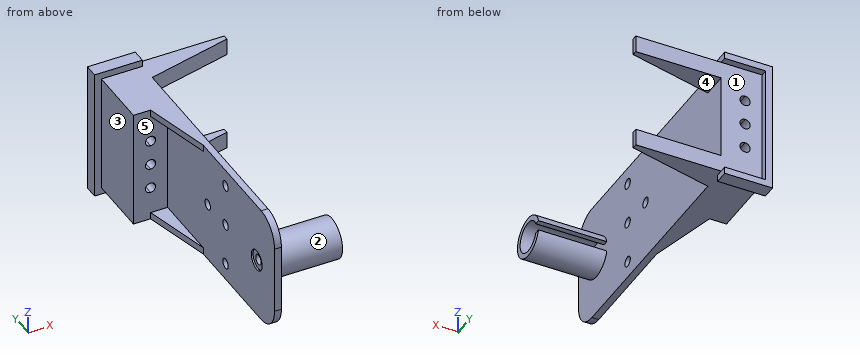
```python
from build123d import *

# Parameters (mm, degrees)
SALIENTE_EXTRUIR1_DEPTH      = 40
SALIENTE_EXTRUIR2_DEPTH      = 4
CROQUIS3_R                   = 3
CORTAR_EXTRUIR1_DEPTH        = 4
CROQUIS4_R                   = 6
CORTAR_EXTRUIR2_DEPTH        = 1
SALIENTE_EXTRUIR3_DEPTH      = 40
SALIENTE_EXTRUIR4_START      = 25
SALIENTE_EXTRUIR4_DEPTH      = 10
SALIENTE_EXTRUIR5_START      = -25
SALIENTE_EXTRUIR5_DEPTH      = 10
SALIENTE_EXTRUIR6_DEPTH      = 4
SALIENTE_EXTRUIR6_DEPTH_BACK = 4
SALIENTE_EXTRUIR6_START      = 140
SALIENTE_EXTRUIR7_START      = 31
SALIENTE_EXTRUIR7_DEPTH      = 4
SALIENTE_EXTRUIR8_START      = -31
SALIENTE_EXTRUIR8_DEPTH      = 4
CORTAR_EXTRUIR3_DEPTH        = 4
CORTAR_EXTRUIR4_DEPTH        = 4
CROQUIS22_R                  = 3
CORTAR_EXTRUIR5_DEPTH        = 4


with BuildPart() as part:
    # Croquis1 → Saliente-Extruir1 (new body)
    with BuildSketch(Plane(origin=(0, 0, 0), x_dir=(0, 0, -1), z_dir=(1, 0, 0))):
        with BuildLine():
            Line((3, 9), (3, 11.618950039))
            ThreePointArc((3, 11.618950039), (0, -12), (-3, 11.618950039))
            Line((-3, 11.618950039), (-3, 9))
            Line((-3, 9), (-3, 8.485281374))
            ThreePointArc((-3, 8.485281374), (0, -9), (3, 8.485281374))
            Line((3, 8.485281374), (3, 9))
        make_face()
    extrude(amount=SALIENTE_EXTRUIR1_DEPTH)

    # Croquis2 → Saliente-Extruir2 (add)
    with BuildSketch(Plane.ZY):
        Polygon((-35, 0), (-35, 140), (35, 140), (35, 0), (35, -20), (-35, -20), align=None)
    extrude(amount=SALIENTE_EXTRUIR2_DEPTH)

    # Croquis3 → Cortar-Extruir1 (cut)
    with BuildSketch(Plane(origin=(0, 0, 0), x_dir=(0, 0, -1), z_dir=(1, 0, 0))):
        Circle(CROQUIS3_R)
    extrude(amount=-CORTAR_EXTRUIR1_DEPTH, mode=Mode.SUBTRACT)

    # Croquis4 → Cortar-Extruir2 (cut)
    with BuildSketch(Plane.ZY.offset(4)):
        Circle(CROQUIS4_R)
    extrude(amount=-CORTAR_EXTRUIR2_DEPTH, mode=Mode.SUBTRACT)

    # Croquis6 → Saliente-Extruir3 (add)
    with BuildSketch(Plane(origin=(0, 140, 0), x_dir=(1, 0, 0), z_dir=(0, 1, 0))):
        with BuildLine():
            Line((-14, 30), (-14, 35))
            Line((-14, 35), (-24, 35))
            Line((-24, 35), (-24, -35))
            Line((-24, -35), (-14, -35))
            Line((-14, -35), (-14, -30))
            Line((-14, -30), (-14, -18))
            ThreePointArc((-14, -18), (-17, -15), (-14, -12))
            Line((-14, -12), (-14, -3))
            ThreePointArc((-14, -3), (-17, 0), (-14, 3))
            Line((-14, 3), (-14, 12))
            ThreePointArc((-14, 12), (-17, 15), (-14, 18))
            Line((-14, 18), (-14, 30))
        make_face()
        with BuildLine():
            Line((-4, 35), (-14, 35))
            Line((-14, 35), (-14, 30))
            Line((-14, 30), (-14, 18))
            ThreePointArc((-14, 18), (-11.878679656, 17.121320344), (-11, 15))
            ThreePointArc((-11, 15), (-11.878679656, 12.878679656), (-14, 12))
            Line((-14, 12), (-14, 3))
            ThreePointArc((-14, 3), (-11.878679656, 2.121320344), (-11, 0))
            ThreePointArc((-11, 0), (-11.878679656, -2.121320344), (-14, -3))
            Line((-14, -3), (-14, -12))
            ThreePointArc((-14, -12), (-11.878679656, -12.878679656), (-11, -15))
            ThreePointArc((-11, -15), (-11.878679656, -17.121320344), (-14, -18))
            Line((-14, -18), (-14, -30))
            Line((-14, -30), (-14, -35))
            Line((-14, -35), (-4, -35))
            Line((-4, -35), (-4, 35))
        make_face()
    extrude(amount=-SALIENTE_EXTRUIR3_DEPTH)

    # Croquis7 → Saliente-Extruir4 (add)
    with BuildSketch(Plane.XY.offset(SALIENTE_EXTRUIR4_START)):
        Polygon((0, 140), (50, 140), (50, 137), (0, 125), align=None)
    extrude(amount=SALIENTE_EXTRUIR4_DEPTH)

    # Croquis8 → Saliente-Extruir5 (add)
    with BuildSketch(Plane.XY.offset(SALIENTE_EXTRUIR5_START)):
        Polygon((0, 140), (50, 140), (50, 137), (0, 125), align=None)
    extrude(amount=-SALIENTE_EXTRUIR5_DEPTH)

    # Croquis9 → Saliente-Extruir6 (add, two sides: drawn at the far end of the back side and taken through both)
    with BuildSketch(Plane(origin=(0, 0, 0), x_dir=(1, 0, 0), z_dir=(0, 1, 0)).offset(SALIENTE_EXTRUIR6_START - SALIENTE_EXTRUIR6_DEPTH_BACK)):
        Polygon((0, 35), (0, 39), (-28, 39), (-28, -39), (-24, -39), (0, -39), (0, -35), (-24, -35), (-24, 35), align=None)
    extrude(amount=SALIENTE_EXTRUIR6_DEPTH + SALIENTE_EXTRUIR6_DEPTH_BACK)

    # Croquis16 → Saliente-Extruir7 (add)
    with BuildSketch(Plane.XY.offset(SALIENTE_EXTRUIR7_START)):
        Polygon((-14, 100), (-4, 60), (-4, 100), align=None)
    extrude(amount=SALIENTE_EXTRUIR7_DEPTH)

    # Croquis17 → Saliente-Extruir8 (add)
    with BuildSketch(Plane.XY.offset(SALIENTE_EXTRUIR8_START)):
        Polygon((-4, 100), (-14, 100), (-4, 60), align=None)
    extrude(amount=-SALIENTE_EXTRUIR8_DEPTH)

    # Croquis19 → Cortar-Extruir3 (cut)
    with BuildSketch(Plane.ZY.offset(4)):
        with BuildLine():
            Line((-35, -20), (-20, -20))
            ThreePointArc((-20, -20), (-30.606601718, -15.606601718), (-35, -5))
            Line((-35, -5), (-35, -20))
        make_face()
        with BuildLine():
            Line((35, -20), (20, -20))
            ThreePointArc((20, -20), (30.606601718, -15.606601718), (35, -5))
            Line((35, -5), (35, -20))
        make_face()
    extrude(amount=-CORTAR_EXTRUIR3_DEPTH, mode=Mode.SUBTRACT)

    # Croquis20 → Cortar-Extruir4 (cut)
    with BuildSketch(Plane.ZY.offset(4)):
        with BuildLine():
            ThreePointArc((-22, 35), (-25, 38), (-28, 35))
            Line((-28, 35), (-22, 35))
        make_face()
        with BuildLine():
            Line((-22, 35), (-28, 35))
            ThreePointArc((-28, 35), (-25, 32), (-22, 35))
        make_face()
        with BuildLine():
            ThreePointArc((3, 35), (0, 38), (-3, 35))
            Line((-3, 35), (3, 35))
        make_face()
        with BuildLine():
            Line((3, 35), (-3, 35))
            ThreePointArc((-3, 35), (0, 32), (3, 35))
        make_face()
        with BuildLine():
            ThreePointArc((22, 35), (25, 32), (28, 35))
            Line((28, 35), (22, 35))
        make_face()
        with BuildLine():
            Line((22, 35), (28, 35))
            ThreePointArc((28, 35), (25, 38), (22, 35))
        make_face()
    extrude(amount=-CORTAR_EXTRUIR4_DEPTH, mode=Mode.SUBTRACT)

    # Croquis22 → Cortar-Extruir5 (cut)
    with BuildSketch(Plane.ZY.offset(4)):
        with Locations((0, 55)):
            Circle(CROQUIS22_R)
    extrude(amount=-CORTAR_EXTRUIR5_DEPTH, mode=Mode.SUBTRACT)


solid = part.part
```
Source: CAD feature listing. Evaluate the final solid. Frame: model axes, mm. Face numbers are marked on the shaded views. A direction names the side the tool comes from. Give positions to 0.01 mm unless a question says otherwise; leave off trailing zeros. Order: outer loops, then holes, each group sorted by start corner. A loop starts at its lowest first (then second) coordinate and runs counter-clockwise, first axis right, second up.
(1) Section query C-C (y = 55). Return the cut outline in (x, z).
(2) Pull-direction query (Z, two-part tool) for the marked faces 1, 2 and 3; classes: +Z half, -Z half, draft (parallel to the pull), parting line (faces both ways), or undercut.
(3) Access query for the marked faces 4 and 5. Directions: +Z, -Z, +X, -X, +Y, -Y. A direction counts if a zero-diameter tool reaches every point of the face in a straight line with its end or side. Return the directions, or none.
(4) Contact query for flat-ended pins moving along their axis: P1, Ø4.5, axis at y = 142, z = -38, coming from the +X side; P2, Ø16, axis at x = -19, z = -4.5, coming from the -Y side; P3, Ø9.5, axis at y = 35, z = 25, coming from the -X side; P4, Ø3.5, axis at y = 35, z = -25, coming from the -X side. Output: stop coordinate, or through.
(5) Material intervals for line 1 along Y through (x, z) = (-1.95, 0); line 2 along Z through (x, y) = (0.5, 127); line 3 along X through (y, z) = (89, -1.5), sorted ascending.
(6) Section query A-A (x = 37.5). Return the cut outline in (y, z), plus the area to 3 significant figures.
(7) Section query D-D (y = 115). Return the cut outline in (x, z).
(8) Section query B-B (y = 35). Return the cut outline in (x, z).
Outcome:
1. outline: (-4, -35) - (0, -35) - (0, -3) - (-4, -3) - close; (-4, 3) - (0, 3) - (0, 35) - (-4, 35) - close
2. face 1: undercut
2. face 2: parting line
2. face 3: draft
3. face 4: +X, +Y, -Y
3. face 5: -X, -Y
4. P1: stops at x = 0
4. P2: stops at y = 100
4. P3: stops at x = -4
4. P4: passes through
5. line 1: y = -20 to -3, 3 to 32, 38 to 52, 58 to 140
5. line 2: z = -35 to -25, 25 to 35
5. line 3: x = -4 to 0
6. outline: (8.49, -3) arc R9 cw (long way) to (8.49, 3) - (11.62, 3) arc R12 ccw (long way) to (11.62, -3) - close; (134, -35) - (140, -35) - (140, -25) - (134, -25) - close; (134, 25) - (140, 25) - (140, 35) - (134, 35) - close
6. area: 300 mm2
7. outline: (-24, -35) - (0, -35) - (0, 35) - (-24, 35) - close; hole circle Ø6 at (-14, -15); hole circle Ø6 at (-14, 0); hole circle Ø6 at (-14, 15)
8. outline: (-4, -35) - (0, -35) - (0, -28) - (-4, -28) - close; (-4, -22) - (0, -22) - (0, -3) - (-4, -3) - close; (-4, 3) - (0, 3) - (0, 22) - (-4, 22) - close; (-4, 28) - (0, 28) - (0, 35) - (-4, 35) - close
